For this review, use the dimensioned drawing (mm, ordinates from the lowest corner) and the shaded views. A direction names the side the tool comes from. Give positions to 0.01 mm unless a question says otherwise; leave off trailing zeros. Write each loop counter-clockwise with the first axis right and the second up, starting at its lowest first coordinate (ties: lowest second). Pieces come first, ordered by that corner, then holes. Notation, with made-up numbers: (75.5, -14.5) - (118.5, -14.5) arc R13 ccw to (118.5, -7.5) - close; hole circle Ø4 at (-6, 32). An arc over 180 degrees is marked (long way). One line per question, with ' | ' between items. Start each with the question number.
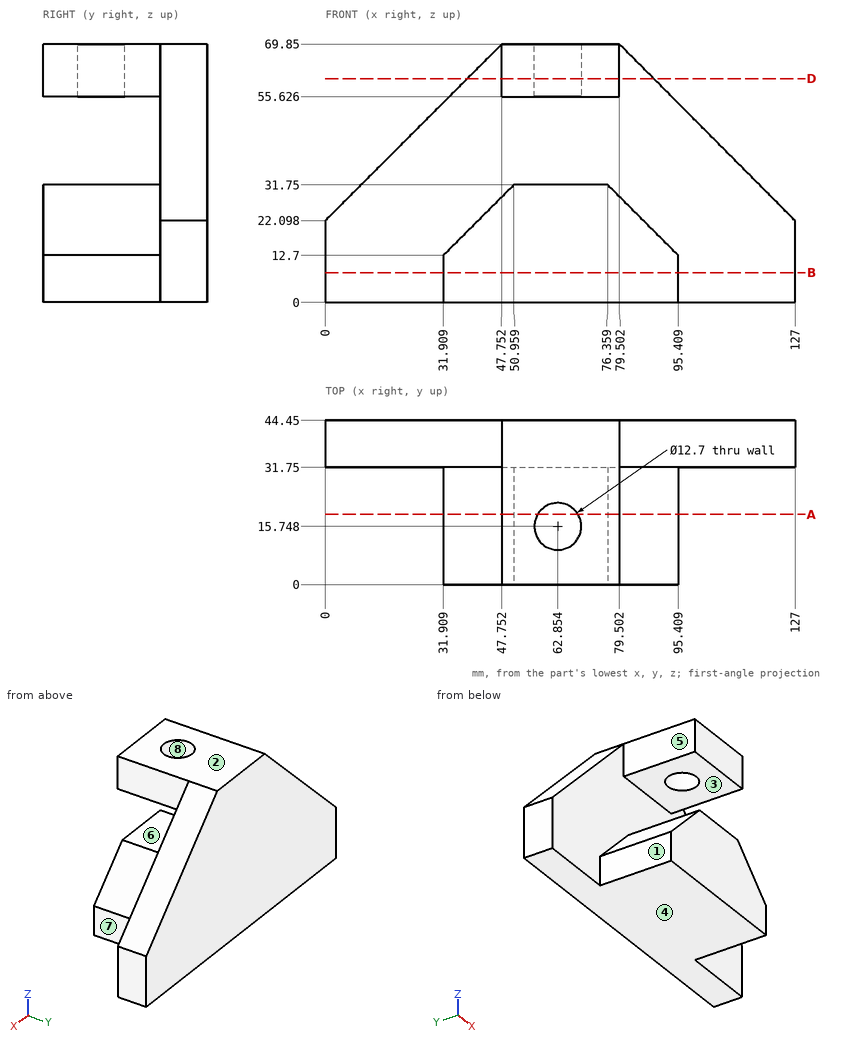
Item 1: Take a section at B-B (z = 8). Give the boundary of the cut face in (x, y), plus the area to 3 significant figures.
Item 2: For probe 1 along Z at (x, y) = (61, 23.5); probe 2 along Y at (x, z) = (23.5, 16); probe 3 along X at (y, z) = (14.5, 7.5), list the stretches that pass through material, from the lowest coordinate up.
Item 3: Clearance check with flat-ended pins moving along their axes: P1, Ø4.5, axis at y = 9, z = 63, coming from the -X side; P2, Ø14, axis at y = 12, z = 8, coming from the +X side; P3, Ø1, axis at x = 56.5, z = 49.5, coming from the -Y side. State where each tip first meets the part, or that it passes through.
Item 4: Machinability: for the marked faces 5, 6, 7 and 8, which of the approach directions +Z, -Z, +X, -X, +Y, -Y give a long, thin tool a straight path to every point of the face, cutting with its end or side? Answer none if there is none.
Item 5: Take a section at D-D (z = 60.5). Give the boundary of the cut face in (x, y), plus the area to 3 significant figures.
Item 6: The part is to be moulded in two halves that separate along Z. For the marked faces 1, 2, 3 and 4, say which applies: +Z half, -Z half, draft (parallel to the pull), parting line (faces both ways), or undercut.
Item 7: Take a section at A-A (y = 19). Give the boundary of the cut face in (x, z), plus the area to 3 significant figures.
Check sheet entries:
1) outline: (0, 31.75) - (31.91, 31.75) - (31.91, 0) - (95.41, 0) - (95.41, 31.75) - (127, 31.75) - (127, 44.45) - (0, 44.45) - close | area: 3,630 mm^2
2) probe 1: z = 0 to 31.75, 55.63 to 69.85 | probe 2: y = 31.75 to 44.45 | probe 3: x = 31.91 to 95.41
3) P1: stops at x = 47.75 | P2: stops at x = 95.41 | P3: stops at y = 31.75
4) face 5: +Z, -X, -Y | face 6: +X, -X, -Y | face 7: +Z, -Z, +X, -Y | face 8: +Z
5) outline: (38.4, 31.75) - (47.75, 31.75) - (47.75, 0) - (79.5, 0) - (79.5, 31.75) - (88.8, 31.75) - (88.8, 44.45) - (38.4, 44.45) - close; hole circle Ø12.7 at (62.85, 15.75) | area: 1,520 mm^2
6) face 1: draft | face 2: +Z half | face 3: undercut | face 4: -Z half
7) outline: (31.91, 0) - (95.41, 0) - (95.41, 12.7) - (76.36, 31.75) - (50.96, 31.75) - (31.91, 12.7) - close; (47.75, 55.63) - (57.4, 55.63) - (57.4, 69.85) - (47.75, 69.85) - close; (68.31, 55.63) - (79.5, 55.63) - (79.5, 69.85) - (68.31, 69.85) - close | area: 1,950 mm^2
